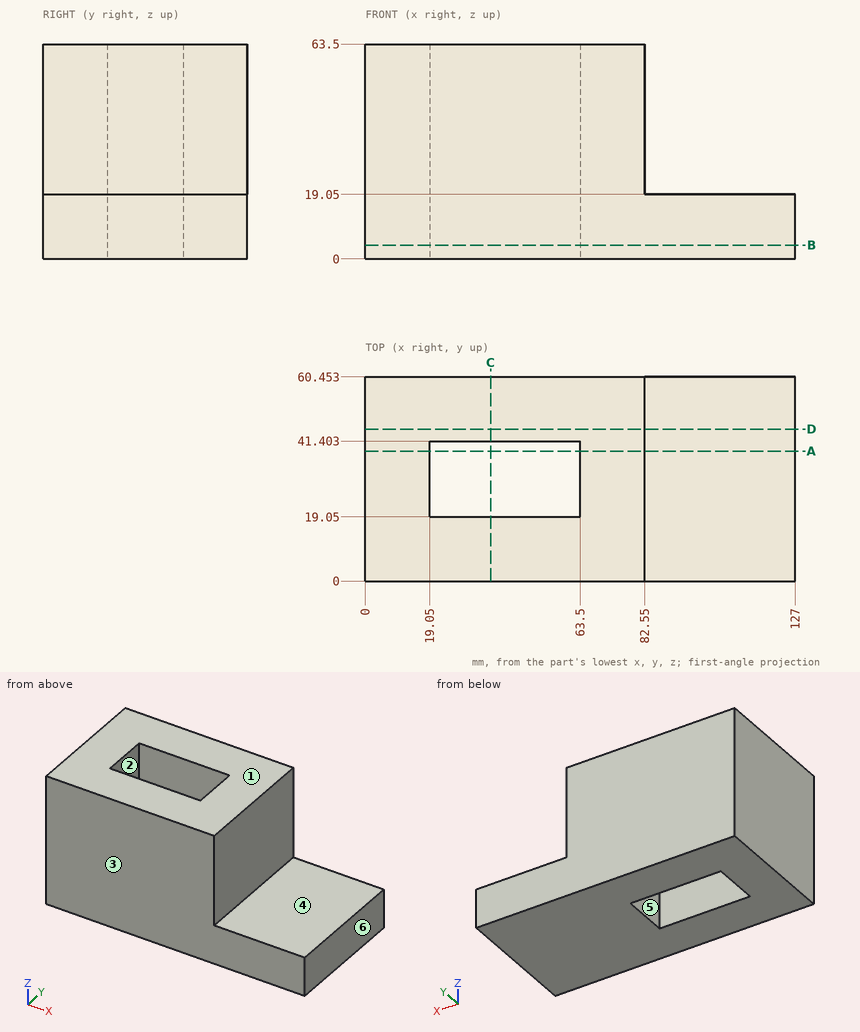
Geometry check sheet. Reference: drawing and pictorial views, mm from the part's lowest x, y, z. A direction names the side the tool comes from. Round coordinates to 2 decimals unless told otherwise and drop trailing zeros. Order: outer loops, then holes, each group sorted by start corner. A loop starts at its lowest first (then second) coordinate and runs counter-clockwise, first axis right, second up. Notation, with made-up numbers: (3, 20) - (41, 20) arc R23 cw to (41, 59) - close; hole circle Ø1 at (11, -10.75). An arc over 180 degrees is marked (long way). Use a Markdown table: item, result. Add a question column.
1) Gauge pin test, flat ends, axial feed: P1, Ø13.5, axis at x = 95, y = 41.5, coming from the +Z side; P2, Ø18, axis at y = 34.5, z = 36.5, coming from the +X side. Record the tip position at first contact, or that the pin passes through.
2) Mould release check, pull along Y, two halves, no side actions. Record for the marked faces 1, 2 and 3: released by +Y, released by -Y, zero draft, split by the parting line, or undercut.
3) Section check B-B (z = 4). Record the cut outline in (x, y).
4) Set-up check for the marked faces 4, 5 and 6: record each of +Z, -Z, +X, -X, +Y, -Y from which the full face is reachable in a straight line by a thin tool's end or side.
5) Section check A-A (y = 38.5). Record the cut outline in (x, z), then the cut area to 3 significant figures.
6) Section check C-C (x = 37). Record the cut outline in (y, z), then the cut area to 3 significant figures.
7) Thickness scan on line 1 along Y through (x, z) = (38, 31); line 2 along X through (y, z) = (35.5, 23); line 3 along X through (y, z) = (30, 15.5). Record the ranges inside material, lowest first.
8) Section check D-D (y = 45). Record the cut outline in (x, z).
Established:
| question | item | result |
|---|---|---|
| 1 | P1 | z = 19.05 |
| 1 | P2 | x = 82.55 |
| 2 | face 1 | zero draft |
| 2 | face 2 | undercut |
| 2 | face 3 | released by -Y |
| 3 | outline | (0, 0) - (127, 0) - (127, 60.45) - (0, 60.45) - close; hole (19.05, 19.05) - (63.5, 19.05) - (63.5, 41.4) - (19.05, 41.4) - close |
| 4 | face 4 | +Z, +X, +Y, -Y |
| 4 | face 5 | +Z, -Z |
| 4 | face 6 | +Z, -Z, +X, +Y, -Y |
| 5 | outline | (0, 0) - (19.05, 0) - (19.05, 63.5) - (0, 63.5) - close; (63.5, 0) - (127, 0) - (127, 19.05) - (82.55, 19.05) - (82.55, 63.5) - (63.5, 63.5) - close |
| 5 | area | 3,270 mm2 |
| 6 | outline | (0, 0) - (19.05, 0) - (19.05, 63.5) - (0, 63.5) - close; (41.4, 0) - (60.45, 0) - (60.45, 63.5) - (41.4, 63.5) - close |
| 6 | area | 2,420 mm2 |
| 7 | line 1 | 0 to 19.05, 41.4 to 60.45 |
| 7 | line 2 | 0 to 19.05, 63.5 to 82.55 |
| 7 | line 3 | 0 to 19.05, 63.5 to 127 |
| 8 | outline | (0, 0) - (127, 0) - (127, 19.05) - (82.55, 19.05) - (82.55, 63.5) - (0, 63.5) - close |
